Part model, mm, in its own coordinate system. A direction names the side the tool comes from. Round coordinates to 2 decimals unless told otherwise and drop trailing zeros. Loops run counter-clockwise (first coordinate to the right, second up) from the corner with the lowest first, then second, coordinate; pieces in that order, holes last. Notation, with made-up numbers: M -27.5,41.25 L 6.5,41.25 A32 cw 6.5,76.25 Z; hole C 47.25,84.5 d11. An arc over 180 degrees is marked long. Put each result on its own line as item: value. Start each with the question number.
1) Slice it at B-B on y = -15. Give the cut face in (x, z) (3 decimals).
2) Slice it at A-A on x = 0. Give the cut face in (y, z) (3 decimals), then the cut area to 3 significant figures.
3) Slice it at C-C on z = 10. Give the cut face in (x, y), then the cut area to 3 significant figures.
4) Pull direction Y, two halves, no side cores. Call faces 1 (the cylindrical face through (-6.344, -12.421, -35.208)), 2 (the flat face through (5.5, 0, 28.4)), 3 (the flat face through (5.5, -25.4, 28.4)): +Y half, -Y half, draft (parallel to the pull), parting line (faces both ways), or undercut.
5) Which spindle directions (+Z, -Z, +X, -X, +Y, -Y) get a long thin tool onto all of the face, cutting with end or side? Do faces 4 (the flat face through (1, -8, 32.385)), 5 (the flat face through (1, -8, -32.385)), 6 (the cylindrical face through (-4.44, -12.5, -30.27)). Say none if no direction does.
6) Slice it at D-D on x = 24. Give the cut face in (y, z).
7) Drop flat-ended pins along their axis: pin 1 Ø5 at (y, z) = (-10, -29) entering from +X; pin 2 Ø4 at (x, y) = (-3, -13.5) entering from -Z (3 decimals); pin 3 Ø10 at (x, y) = (0, -12.7) entering from +Z (3 decimals); pin 4 Ø6 at (x, z) = (4.5, -24.5) entering from -Y. Give the stop position or say it passes through.
8) Probe line 1 along Y through (x, z) = (0, 29.7) (3 decimals); line 2 along Y through (x, z) = (0, -35); line 3 along Z through (x, y) = (-8, -14.5). List the from-to ranges inside material, lowest first.
```python
from build123d import *

# Parameters (mm, degrees)
F0_R     = 38.1
F0_R_2   = 28.575
F1_DEPTH = 25.4
F2_R     = 4.445
F3_DEPTH = 38.1
F5_R     = 6.35
F5_R_2   = 4.445
F6_DEPTH = 25.4
F8_R     = 6.35
F8_R_2   = 4.445
F9_DEPTH = 25.4


with BuildPart() as f1:
    # F0 (on Front) → F1 (new body)
    with BuildSketch(Plane.XZ):
        Circle(F0_R)
        Circle(F0_R_2, mode=Mode.SUBTRACT)
    extrude(amount=F1_DEPTH)

    # F2 (on Top) → F3 (cut, symmetric)
    with BuildSketch(Plane.XY):
        with Locations((0, -12.7)):
            Circle(F2_R)
    extrude(amount=F3_DEPTH, both=True, mode=Mode.SUBTRACT)

    # F5 (on offset) → F6 (cut)
    with BuildSketch(Plane.XY.offset(32.385)):
        with Locations((0, -12.7)):
            Circle(F5_R)
        with Locations((0, -12.7)):
            Circle(F5_R_2, mode=Mode.SUBTRACT)
    extrude(amount=F6_DEPTH, mode=Mode.SUBTRACT)

    # F8 (on offset) → F9 (cut)
    with BuildSketch(Plane.XY.offset(-32.385)):
        with Locations((0, -12.7)):
            Circle(F8_R)
        with Locations((0, -12.7)):
            Circle(F8_R_2, mode=Mode.SUBTRACT)
    extrude(amount=-F9_DEPTH, mode=Mode.SUBTRACT)


solid = f1.part
```
Recorded:
1. outline: M -5.919,-37.637 L -5.919,-32.385 L -3.804,-32.385 L -3.804,-28.321 A28.575 cw -3.804,28.321 L -3.804,32.385 L -5.919,32.385 L -5.919,37.637 A38.1 ccw Z; M 3.804,-32.385 L 5.919,-32.385 L 5.919,-37.637 A38.1 ccw 5.919,37.637 L 5.919,32.385 L 3.804,32.385 L 3.804,28.321 A28.575 cw 3.804,-28.321 Z
2. outline: M -25.4,-38.1 L -19.05,-38.1 L -19.05,-32.385 L -17.145,-32.385 L -17.145,-28.575 L -25.4,-28.575 Z; M -25.4,28.575 L -17.145,28.575 L -17.145,32.385 L -19.05,32.385 L -19.05,38.1 L -25.4,38.1 Z; M -8.255,-32.385 L -6.35,-32.385 L -6.35,-38.1 L 0,-38.1 L 0,-28.575 L -8.255,-28.575 Z; M -8.255,28.575 L 0,28.575 L 0,38.1 L -6.35,38.1 L -6.35,32.385 L -8.255,32.385 Z
2. area: 271 mm2
3. outline: M -36.76,-25.4 L -26.77,-25.4 L -26.77,0 L -36.76,0 Z; M 26.77,-25.4 L 36.76,-25.4 L 36.76,0 L 26.77,0 Z
3. area: 508 mm2
4. face 1: undercut
4. face 2: +Y half
4. face 3: -Y half
5. face 4: +Z
5. face 5: -Z
5. face 6: +Z, -Z
6. outline: M -25.4,-29.59 L 0,-29.59 L 0,-15.51 L -25.4,-15.51 Z; M -25.4,15.51 L 0,15.51 L 0,29.59 L -25.4,29.59 Z
7. pin 1: stops at x = 27.37
7. pin 2: stops at z = -32.385
7. pin 3: stops at z = 32.385
7. pin 4: passes through
8. line 1: y = -25.4 to -17.145, -8.255 to 0
8. line 2: y = -25.4 to -19.05, -6.35 to 0
8. line 3: z = -37.25 to -27.43, 27.43 to 37.25
